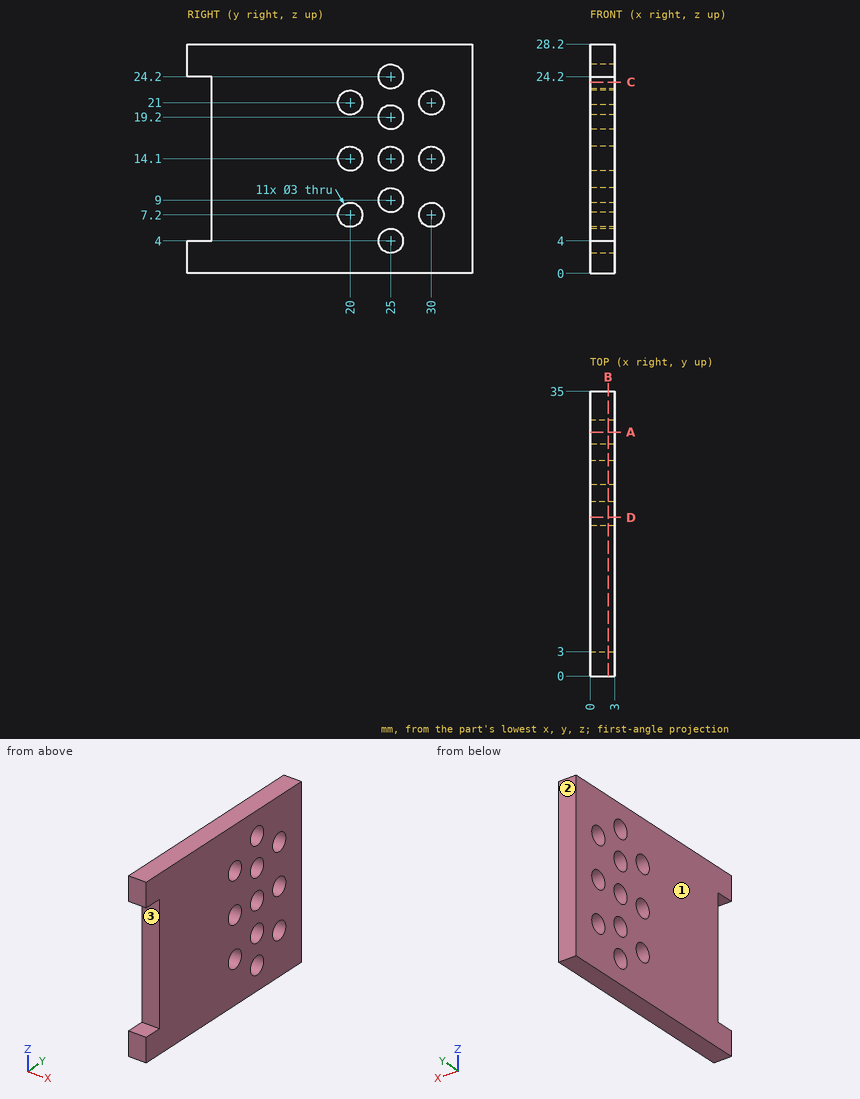
Drawing for the job (mm, zero at the part's lowest x, y, z). Give positions to 0.01 mm unless a question says otherwise; leave off trailing zeros. Loops run counter-clockwise (first coordinate to the right, second up) from the corner with the lowest first, then second, coordinate; pieces in that order, holes last.
1) Band-saw the part on A-A on y = 30. List the corners of the cut face in (x, z).
Values follow:
outline: (0, 0) - (3, 0) - (3, 5.7) - (0, 5.7) - close; (0, 8.7) - (3, 8.7) - (3, 12.6) - (0, 12.6) - close; (0, 15.6) - (3, 15.6) - (3, 19.5) - (0, 19.5) - close; (0, 22.5) - (3, 22.5) - (3, 28.2) - (0, 28.2) - close
2) Band-saw the part on C-C on z = 23.5. List the corners of the cut face in (x, y), then the cut area to 3 significant figures.
Values follow:
outline: (0, 3) - (3, 3) - (3, 23.67) - (0, 23.67) - close; (0, 26.33) - (3, 26.33) - (3, 35) - (0, 35) - close
area: 88.0 mm2
3) Drop a flat-ended pin along its axis: P1, Ø1.5, axis at x = 2.5, z = 21, coming from the -Y side. Give the stop position or say it passes through.
Values follow:
P1: stops at y = 3
4) Band-saw the part on B-B on x = 2.2. State how many separate pieces and enclosed holes the cut face has, then the cut area to 3 significant figures.
Values follow:
separate pieces: 1
enclosed holes: 11
area: 849 mm2
5) Two-plate mould, pull along Y, no slides. Class the marked faces 1, 2 and 3: released by +Y, released by -Y, zero draft, split by the parting line, or undercut.
Values follow:
face 1: zero draft
face 2: released by +Y
face 3: released by -Y
6) Band-saw the part on D-D on y = 19.5. List the corners of the cut face in (x, z), then the cut area to 3 significant figures.
Values follow:
outline: (0, 0) - (3, 0) - (3, 5.79) - (0, 5.79) - close; (0, 8.61) - (3, 8.61) - (3, 12.69) - (0, 12.69) - close; (0, 15.51) - (3, 15.51) - (3, 19.59) - (0, 19.59) - close; (0, 22.41) - (3, 22.41) - (3, 28.2) - (0, 28.2) - close
area: 59.1 mm2
7) Probe line 1 along Z through (x, y) = (1.65, 30); line 2 along Y through (x, z) = (2.3, 13.25); line 3 along Y through (x, z) = (1.5, 20.25). List the from-to ranges inside material, lowest first.
Values follow:
line 1: z = 0 to 5.7, 8.7 to 12.6, 15.6 to 19.5, 22.5 to 28.2
line 2: y = 3 to 18.76, 21.24 to 23.76, 26.24 to 28.76, 31.24 to 35
line 3: y = 3 to 18.7, 21.3 to 23.93, 26.07 to 28.7, 31.3 to 35
